```python
from build123d import *

# Parameters (mm, degrees)
SKETCH_1_R               = 12.5
EXTRUDE_1_DEPTH          = 1.5
CUT_EXTRUDE_1_DEPTH      = 2
SKETCH_3_R               = 1.05
CUT_EXTRUDE_2_DEPTH      = 22
EXTRUDE_START            = -1.5
SKETCH_4_R               = 3
EXTRUDE_2_DEPTH          = 3
PATTERN_CIRCULAR_1_COUNT = 18
SKETCH_5_R               = 1.05
CUT_EXTRUDE_3_DEPTH      = 23


with BuildPart() as part:
    # 스케치1 → 보스-돌출1 (new body)
    with BuildSketch(Plane(origin=(0, 0, 0), x_dir=(1, 0, 0), z_dir=(0, 1, 0))):
        Circle(SKETCH_1_R)
    extrude(amount=EXTRUDE_1_DEPTH)

    # 스케치2 → 컷-돌출1 (cut)
    with BuildSketch(Plane(origin=(0, 1.5, 0), x_dir=(1, 0, 0), z_dir=(0, 1, 0))):
        Polygon((-0.75, 6.959705454), (0.444838448, 6.985851326), (1.05510653, 10.446853603), (-0.75, 10.473180033), align=None)
    cut_extrude_1 = extrude(amount=-CUT_EXTRUDE_1_DEPTH, mode=Mode.SUBTRACT)

    # 스케치3 → 컷-돌출2 (cut)
    with BuildSketch(Plane(origin=(0, 1.5, 0), x_dir=(1, 0, 0), z_dir=(0, 1, 0))):
        Circle(SKETCH_3_R)
    extrude(amount=-CUT_EXTRUDE_2_DEPTH, mode=Mode.SUBTRACT)

    # 스케치4 → 보스-돌출2 (add)
    with BuildSketch(Plane(origin=(0, 1.5, 0), x_dir=(1, 0, 0), z_dir=(0, 1, 0)).offset(EXTRUDE_START)):
        Circle(SKETCH_4_R)
    extrude(amount=-EXTRUDE_2_DEPTH)

    # 원형 패턴1: 컷-돌출1 ×18 about axis
    pattern_circular_1_axis = Axis((0, 0, 0), (0, 1, 0))
    for i in range(1, PATTERN_CIRCULAR_1_COUNT):
        add(cut_extrude_1.rotate(pattern_circular_1_axis, i * 360 / PATTERN_CIRCULAR_1_COUNT), mode=Mode.SUBTRACT)

    # 스케치5 → 컷-돌출3 (cut)
    with BuildSketch(Plane(origin=(0, 1.5, 0), x_dir=(1, 0, 0), z_dir=(0, 1, 0))):
        Circle(SKETCH_5_R)
    extrude(amount=-CUT_EXTRUDE_3_DEPTH, mode=Mode.SUBTRACT)


solid = part.part
```
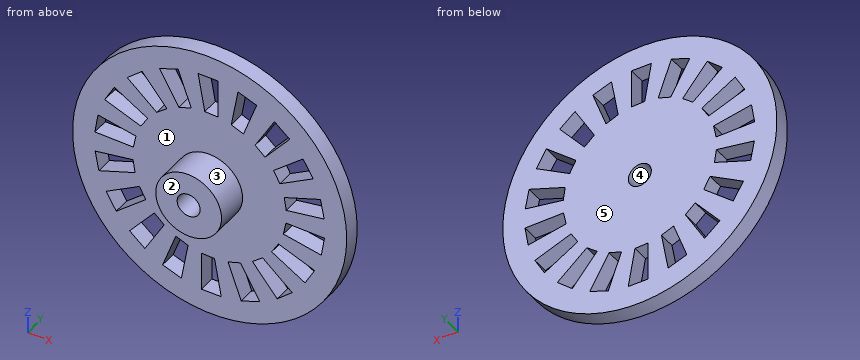
Part model, mm, in its own coordinate system. Face numbers are marked on the shaded views. A direction names the side the tool comes from. Coordinates: 2 decimals unless noted, no trailing zeros. Write each loop counter-clockwise with the first axis right and the second up, starting at its lowest first coordinate (ties: lowest second). Pieces come first, ordered by that corner, then holes.
Item 1: Slice it at A-A (z = 0). Write the cut outline in (x, y).
Item 2: Mould opens along Z. For the marked faces 3, 4 and 5 say: released by +Z, released by -Z, zero draft, split by the parting line, or undercut.
Item 3: Probe line 1 (X direction, y = -2.1, z = 0); line 2 (Y direction, x = -5, z = -9.5). List the from-to ranges inside material, lowest first.
Item 4: Slice it at D-D (y = -0.55). Write the cut outline in (x, z), and give its area (3 significant figures).
Item 5: Slice it at C-C (z = 3.5). Write the cut outline in (x, y), and give its area (3 significant figures).
Item 6: Pin check, flat tips, straight feed: pin 1 (1.2 mm diameter, centred on y = 0.5, z = -8.5, fed in from +X); pin 2 (1.2 mm diameter, centred on y = 0.5, z = 9, fed in from -X); pin 3 (1.2 mm diameter, centred on x = -8.5, y = 1, fed in from +Z). Stop position of each tip, or through.
Item 7: Slice it at B-B (x = 0). Write the cut outline in (y, z).
Item 8: Which spindle directions (+Z, -Z, +X, -X, +Y, -Y) get a long thin tool onto all of the face, cutting with end or side? Do the marked faces 1 and 2. Say none if no direction does.
Results found:
1. outline: (-12.5, 0) - (-3, 0) - (-3, -3) - (-1.05, -3) - (-1.05, 1.5) - (-12.5, 1.5) - close; (1.05, -3) - (3, -3) - (3, 0) - (12.5, 0) - (12.5, 1.5) - (1.05, 1.5) - close
2. face 3: split by the parting line
2. face 4: undercut
2. face 5: zero draft
3. line 1: x = -3 to -1.05, 1.05 to 3
3. line 2: y = 0 to 1.5
4. outline: circle Ø6 at (0, 0); hole circle Ø2.1 at (0, 0)
4. area: 24.8 mm2
5. outline: (-12, 0) - (-7.35, 0) - (-7.35, 1.5) - (-12, 1.5) - close; (-6.03, 0) - (6.03, 0) - (6.03, 1.5) - (-6.03, 1.5) - close; (7.56, 0) - (12, 0) - (12, 1.5) - (7.56, 1.5) - close
5. area: 31.7 mm2
6. pin 1: stops at x = 9.69
6. pin 2: stops at x = -9.26
6. pin 3: stops at z = 9.69
7. outline: (-3, -3) - (0, -3) - (0, -6.98) - (1.5, -6.98) - (1.5, -1.05) - (-3, -1.05) - close; (-3, 1.05) - (1.5, 1.05) - (1.5, 6.98) - (0, 6.98) - (0, 3) - (-3, 3) - close; (0, -12.5) - (1.5, -12.5) - (1.5, -10.46) - (0, -10.46) - close; (0, 10.46) - (1.5, 10.46) - (1.5, 12.5) - (0, 12.5) - close
8. face 1: -Y
8. face 2: +Z, -Z, +X, -X, -Y
